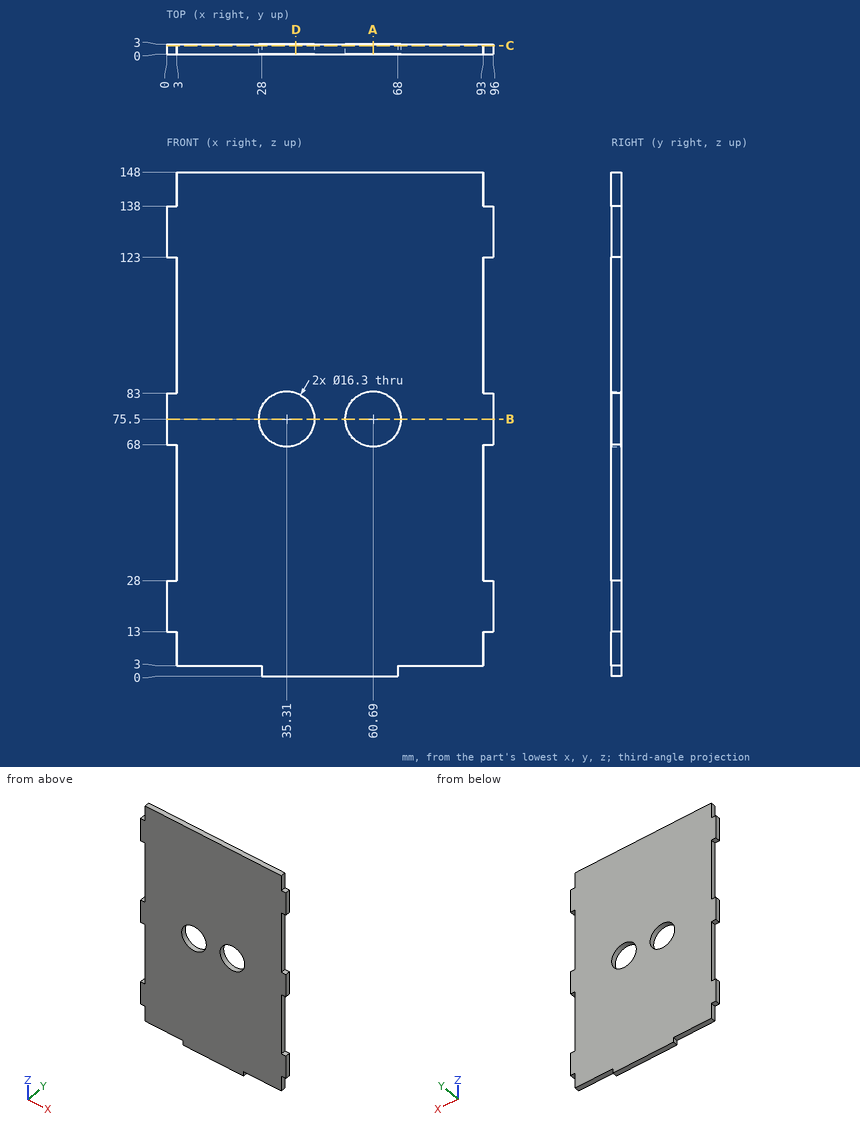
Here's the drawing with two shaded views (mm, measured from the low corner). I have some questions. Give positions to 0.01 mm unless a question says otherwise; leave off trailing zeros. Write each loop counter-clockwise with the first axis right and the second up, starting at its lowest first coordinate (ties: lowest second). Pieces come first, ordered by that corner, then holes. Notation, with made-up numbers: (-13, -12) - (29, -12) arc R30 cw to (29, 17) - close; hole circle Ø3 at (-21, -29). An arc over 180 degrees is marked (long way). One line per item, written item: value. Start each with the question number.
Item 1: I'm going to push flat-ended pins straight in: pin 1 (1.5 mm diameter, centred on x = 78, y = 1.5, fed in from -Z); pin 2 (0.9 mm diameter, centred on y = 1, z = 8.5, fed in from +X); pin 3 (1.5 mm diameter, centred on x = 94, y = 2, fed in from -Z). Where does each tip first touch, or does it pass through?
Item 2: Imagine slicing it at A-A, the plane x = 60.69. List the corners of the cut face in (y, z) for me, and give its area (3 significant figures).
Item 3: Please list where these lines run through material, in increasing order: line 1 (X direction, y = 1.95, z = 75.5); line 2 (X direction, y = 2.45, z = 76.5); line 3 (Z direction, x = 60.69, y = 2.1). Write a range as from..to.
Item 4: Imagine slicing it at C-C, the plane y = 2.5. Give the number of separate pieces and of enclosed holes in the cut face, and give its area (3 significant figures).
Item 5: Imagine slicing it at D-D, the plane x = 38. List the corners of the cut face in (y, z) for me.
Item 6: Imagine slicing it at B-B, the plane z = 75.5. List the corners of the cut face in (x, y) for me.
Geometry says:
1. pin 1: z = 3
1. pin 2: x = 93
1. pin 3: z = 13
2. outline: (0, 0) - (3, 0) - (3, 67.35) - (0, 67.35) - close; (0, 83.65) - (3, 83.65) - (3, 148) - (0, 148) - close
2. area: 395 mm^2
3. line 1: 0..27.16, 43.46..52.54, 68.84..96
3. line 2: 0..27.22, 43.4..52.6, 68.78..96
3. line 3: 0..67.35, 83.65..148
4. separate pieces: 1
4. enclosed holes: 2
4. area: 13,000 mm^2
5. outline: (0, 0) - (3, 0) - (3, 67.81) - (0, 67.81) - close; (0, 83.19) - (3, 83.19) - (3, 148) - (0, 148) - close
6. outline: (0, 0) - (27.16, 0) - (27.16, 3) - (0, 3) - close; (43.46, 0) - (52.54, 0) - (52.54, 3) - (43.46, 3) - close; (68.84, 0) - (96, 0) - (96, 3) - (68.84, 3) - close
